```python
from build123d import *

# Parameters (mm, degrees)
PAD_DEPTH    = 2
PAD001_DEPTH = 1
SKETCH002_R  = 1.3
POCKET_DEPTH = 1.001
FILLET_R     = 1
FILLET001_R  = 0.3
FILLET002_R  = 0.3
CHAMFER_SIZE = 0.3


with BuildPart() as part:
    # Sketch → Pad (new body)
    with BuildSketch(Plane.XY):
        with BuildLine():
            ThreePointArc((2, -3.464102), (0, 4), (-2, -3.464102))
            Line((-2, -24), (-2, -3.464102))
            Line((2, -24), (-2, -24))
            Line((2, -3.464102), (2, -24))
        make_face()
        Polygon((0, 2.367136), (-2.05, 1.183568), (-2.05, -1.183568), (0, -2.367136), (2.05, -1.183568), (2.05, 1.183568), align=None, mode=Mode.SUBTRACT)
    extrude(amount=PAD_DEPTH)

    # Sketch001 (on Face11 of Pad) → Pad001 (join)
    with BuildSketch(Plane(origin=(0, 0, 0), x_dir=(1, 0, 0), z_dir=(0, 0, -1))):
        with BuildLine():
            ThreePointArc((-2, 3.464102), (0, -4), (2, 3.464102))
            Line((2, 3.464102), (2, 24))
            Line((2, 24), (-2, 24))
            Line((-2, 24), (-2, 3.464102))
        make_face()
    extrude(amount=PAD001_DEPTH)

    # Sketch002 (on Face17 of Pad001) → Pocket (cut, through all)
    with BuildSketch(Plane.XY):
        Circle(SKETCH002_R)
    extrude(amount=-POCKET_DEPTH, mode=Mode.SUBTRACT)

    # Fillet
    fillet_edges = [part.edges().sort_by_distance(p)[0] for p in [
        (2, -13.732051, 2),
        (0, -24, 2),
        (-2, -13.732051, 2),
        (0, 4, 2),
    ]]
    fillet(fillet_edges, radius=FILLET_R)

    # Fillet001
    fillet001_edges = [part.edges().sort_by_distance(p)[0] for p in [
        (2, -24, 0.5),
        (2, -24, -0.5),
    ]]
    fillet(fillet001_edges, radius=FILLET001_R)

    # Fillet002
    fillet002_edges = [part.edges().sort_by_distance(p)[0] for p in [
        (-2, -24, 0.5),
        (-2, -24, -0.5),
    ]]
    fillet(fillet002_edges, radius=FILLET002_R)

    # Chamfer
    chamfer_edges = [part.edges().sort_by_distance(p)[0] for p in [
        (-2.05, 0, 2),
        (-1.025, 1.775352, 2),
        (1.025, 1.775352, 2),
        (2.05, 0, 2),
        (1.025, -1.775352, 2),
        (-1.025, -1.775352, 2),
    ]]
    chamfer(chamfer_edges, length=CHAMFER_SIZE)


solid = part.part
```
Design review of the part built by this model. Coordinates are the model's own, in mm. A direction names the side the tool comes from. Coordinates: 2 decimals unless noted, no trailing zeros. Order: outer loops, then holes, each group sorted by start corner. A loop starts at its lowest first (then second) coordinate and runs counter-clockwise, first axis right, second up. Notation, with made-up numbers: M -28.75,-18.5 L 14.25,-18.5 A13 ccw 14.25,1.5 Z; hole C 40,21 d5. An arc over 180 degrees is marked long. Answer as a JSON object with one key per item and string values. Group by question number.
1) Add section A-A, the plane z = -0.4. Write out the cut boundary in (x, y).
2) Wall thickness on L1, parallel to Y at x = 0, z = -0.6; L2, parallel to Y at x = 0.5, z = 0.5; L3, parallel to X at y = -21, z = 0.85: over which ranges is each line inside the solid? List them lowest first.
3) For pin 1 (1.6 mm diameter, centred on y = -14.5, z = 0.5, fed in from +X); pin 2 (1 mm diameter, centred on y = -9.5, z = 0, fed in from -X); pin 3 (2 mm diameter, centred on x = 0, y = 0, fed in from +Z), all flat-tipped, find the tip position at first contact; note any pin that passes through.
4) Mouldability with a two-part tool opening along X and no side actions: class faces 1 (the flat face through (0, -10, -1)), 2 (the flat face through (1.039, 1.767, 0.838)), 3 (the cylindrical face through (1.715, -13.41, 1.699)), 4 (the flat face through (-2, -14, 0)) as pulls with the +X half, pulls with the -X half, needs draft (parallel to the pull), parting line crosses it, or undercut.
5) Tool access review of faces 5 (the flat face through (0, -10, 2)), 6 (the cylindrical face through (-1.715, -13.118, 1.699)), 7 (the flat face through (2, -13, 0)), 8 (the flat face through (1.083, -1.913, 1.848)): name each direction out of +Z, -Z, +X, -X, +Y, -Y from which nothing blocks a thin tool from reaching the whole face with its end or side.
6) Add section B-B, the plane y = -13.5. Write out the cut boundary in (x, z), then the cut area to 3 significant figures.
Computed values:
{
 "1": {"outline": "M -2,-23.7 A0.3 ccw -1.7,-24 L 1.7,-24 A0.3 ccw 2,-23.7 L 2,-3.46 A4 ccw long -2,-3.46 Z; hole C 0,0 d2.6"},
 "2": {"L1": "y = -24 to -1.3, 1.3 to 4", "L2": "y = -24 to -2.08, 2.08 to 3.97", "L3": "x = -2 to 2"},
 "3": {"pin 1": "stops at x = 2", "pin 2": "stops at x = -2", "pin 3": "passes through"},
 "4": {"face 1": "needs draft", "face 2": "undercut", "face 3": "pulls with the +X half", "face 4": "pulls with the -X half"},
 "5": {"face 5": "+Z, +X, -X, +Y, -Y", "face 6": "+Z, -X, -Y", "face 7": "+Z, -Z, +X, -Y", "face 8": "+Z"},
 "6": {"outline": "M -2,-1 L 2,-1 L 2,1 A1 ccw 1,2 L -1,2 A1 ccw -2,1 Z", "area": "11.6 mm^2"}
}
